Could you check a few things on this model? Use its own coordinates, in mm. A direction names the side the tool comes from. Give positions to 0.01 mm unless a question says otherwise; leave off trailing zeros. Write each loop counter-clockwise with the first axis right and the second up, starting at its lowest first coordinate (ties: lowest second). Pieces come first, ordered by that corner, then holes. Notation, with made-up numbers: (75, 81.5) - (104, 81.5) arc R22 ccw to (104, 119.5) - close; hole circle Ø9 at (42, 0). An arc over 180 degrees is marked (long way). Answer in a Markdown table with one row per item.
from build123d import *

# Parameters (mm, degrees)
F0_W           = 76.2
F0_H           = 76.2
F1_DEPTH       = 24.13
F3_DEPTH       = 76.201
F5_DEPTH       = 76.201
F7_D           = 6.35
F7_CBORE_D     = 12.7
F7_CBORE_DEPTH = 6.35
F8_R           = 5.08
F9_R           = 5.08
F10_R          = 5.08


with BuildPart() as f1:
    # F0 (on Top) → F1 (new body)
    with BuildSketch(Plane.XY):
        with Locations((-38.1, -16.877948)):
            Rectangle(F0_W, F0_H)
    extrude(amount=F1_DEPTH)

    # F2 (on face) → F3 (cut, through all)
    with BuildSketch(Plane.YZ):
        with BuildLine():
            Line((-24.367969, 0), (1.032031, 0))
            ThreePointArc((1.032031, 0), (-11.667969, 12.7), (-24.367969, 0))
        make_face()
    extrude(amount=-F3_DEPTH, mode=Mode.SUBTRACT)

    # F4 (on face) → F5 (cut, through all)
    with BuildSketch(Plane.XZ.offset(54.977948)):
        with BuildLine():
            Line((-57.15, 0), (-19.05, 0))
            ThreePointArc((-19.05, 0), (-38.1, 12.7), (-57.15, 0))
        make_face()
    extrude(amount=-F5_DEPTH, mode=Mode.SUBTRACT)

    # F7 (through all)
    with Locations(Plane.XY.offset(24.13)):
        with Locations((-57.15, -35.927948)):
            CounterBoreHole(F7_D / 2, F7_CBORE_D / 2, F7_CBORE_DEPTH)

    # F8
    f8_edges = [f1.edges().sort_by_distance(p)[0] for p in [
        (-76.2, -16.877948, 24.13),
    ]]
    fillet(f8_edges, radius=F8_R)

    # F9
    f9_edges = [f1.edges().sort_by_distance(p)[0] for p in [
        (-35.56, -54.977948, 24.13),
    ]]
    fillet(f9_edges, radius=F9_R)

    # F10
    f10_edges = [f1.edges().sort_by_distance(p)[0] for p in [
        (0, -14.337948, 24.13),
    ]]
    fillet(f10_edges, radius=F10_R)


solid = f1.part
1) Imagine slicing it at C-C (z = 20). List the corners of the cut face in (x, y) for me, then the cut area to 3 significant figures.
Check values:
| item | result |
|---|---|
| outline | (-76.11, -49.9) arc R4.99 ccw to (-71.12, -54.89) - (-5.08, -54.89) arc R4.99 ccw to (-0.09, -49.9) - (-0.09, 21.22) - (-76.11, 21.22) - close; hole circle Ø12.7 at (-57.15, -35.93) |
| area | 5,650 mm2 |
2) Will these pins go through, and if not, where does the flat tip stop? P1, Ø12, axis at x = -36.5, y = -38, coming from the -Z side; P2, Ø2, axis at x = -48.5, y = 2, coming from the -Z side; P3, Ø4, axis at y = -29, z = 21.5, coming from the -X side.
Check values:
| item | result |
|---|---|
| P1 | stops at z = 11.25 |
| P2 | stops at z = 9.27 |
| P3 | stops at x = -76.18 |
3) Imagine slicing it at D-D (x = -9). List the corners of the cut face in (y, z) for me.
Check values:
| item | result |
|---|---|
| outline | (-54.98, 0) - (-24.37, 0) arc R12.7 cw to (1.03, 0) - (21.22, 0) - (21.22, 24.13) - (-49.9, 24.13) arc R5.08 ccw to (-54.98, 19.05) - close |
4) We'd pull the mould along Y, two halves only. Please class faces 1 (the face through (-60.1, -37.1, 8.8)), 2 (the face through (-1.5, -53.5, 9.7)), 3 (the face through (-1.528, -13.84, 22.681)): +Y half, -Y half, draft (parallel to the pull), parting line (faces both ways), or undercut.
Check values:
| item | result |
|---|---|
| face 1 | undercut |
| face 2 | -Y half |
| face 3 | draft |
5) Imagine slicing it at B-B (x = -40). List the corners of the cut face in (y, z) for me.
Check values:
| item | result |
|---|---|
| outline | (-54.98, 12.61) - (-13.16, 12.61) arc R12.7 cw to (-10.18, 12.61) - (21.22, 12.61) - (21.22, 24.13) - (-49.9, 24.13) arc R5.08 ccw to (-54.98, 19.05) - close |
6) On a 3-axis mill with a long thin cutter (end or side, diameter ignored), from which of +Z, -Z, +X, -X, +Y, -Y can I reach the whole of each face in a straight line? I mean faces 4 (the face through (-60, -34, 17.78)), 5 (the face through (-37.64, -53.53, 22.6)). Say none if no direction works.
Check values:
| item | result |
|---|---|
| face 4 | +Z |
| face 5 | +Z, +X, -X, -Y |
7) If I drill on line 1 (Y direction, x = -57.15, z = 7.5); line 2 (X direction, y = -49, z = 9); line 3 (Y direction, x = -57.15, z = 7.75), over which ranges is the centre line in solid material (lowest first)?
Check values:
| item | result |
|---|---|
| line 1 | y = -54.98 to -39.1, -32.75 to -21.92, -1.42 to 21.22 |
| line 2 | x = -76.2 to -49.89, -26.31 to 0 |
| line 3 | y = -54.98 to -39.1, -32.75 to -21.73, -1.61 to 21.22 |
